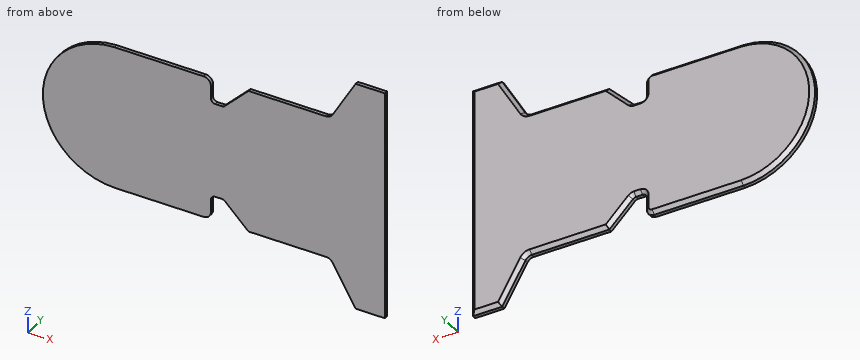
```python
from build123d import *

# Parameters (mm, degrees)
BOSS_EXTRUDE1_DEPTH = 5
CHAMFER1_SIZE       = 2.5


with BuildPart() as part:
    # Sketch1 → Boss-Extrude1 (new body)
    with BuildSketch(Plane(origin=(0, 0, 0), x_dir=(1, 0, 0), z_dir=(0, 1, 0))):
        with BuildLine():
            Line((15.254575611, 35.990242765), (15.254575611, 44.990242765))
            ThreePointArc((15.254575611, 44.990242765), (13.790109517, 48.525776671), (10.254575611, 49.990242765))
            Line((10.254575611, 49.990242765), (-50.745424389, 49.990242765))
            ThreePointArc((-50.745424389, 49.990242765), (-99.757685432, 0), (-50.745424389, -49.990242765))
            Line((-50.745424389, -49.990242765), (10.254575611, -49.990242765))
            ThreePointArc((10.254575611, -49.990242765), (13.790109517, -48.525776671), (15.254575611, -44.990242765))
            Line((15.254575611, -44.990242765), (15.254575611, -35.990242765))
            ThreePointArc((15.254575611, -35.990242765), (16.133255268, -33.868922422), (18.254575611, -32.990242765))
            Line((18.254575611, -32.990242765), (22.711934924, -32.990242765))
            ThreePointArc((22.711934924, -32.990242765), (23.859985221, -33.218604168), (24.833255268, -33.868922422))
            Line((24.833255268, -33.868922422), (40.954575611, -49.990242765))
            Line((40.954575611, -49.990242765), (50.745424389, -49.990242765))
            Line((50.745424389, -49.990242765), (94.067824265, -49.990242765))
            ThreePointArc((94.067824265, -49.990242765), (96.567824265, -50.660115747), (98.397951284, -52.490242765))
            Line((98.397951284, -52.490242765), (114.280717029, -80))
            Line((114.280717029, -80), (134.280717029, -80))
            Line((134.280717029, -80), (134.280717029, 80))
            Line((134.280717029, 80), (114.280717029, 80))
            Line((114.280717029, 80), (98.397951284, 52.490242765))
            ThreePointArc((98.397951284, 52.490242765), (96.567824265, 50.660115747), (94.067824265, 49.990242765))
            Line((94.067824265, 49.990242765), (50.745424389, 49.990242765))
            Line((50.745424389, 49.990242765), (40.954575611, 49.990242765))
            Line((40.954575611, 49.990242765), (24.833255268, 33.868922422))
            ThreePointArc((24.833255268, 33.868922422), (23.859985221, 33.218604168), (22.711934924, 32.990242765))
            Line((22.711934924, 32.990242765), (18.254575611, 32.990242765))
            ThreePointArc((18.254575611, 32.990242765), (16.133255268, 33.868922422), (15.254575611, 35.990242765))
        make_face()
    extrude(amount=BOSS_EXTRUDE1_DEPTH)

    # Chamfer1
    chamfer1_edges = [part.edges().sort_by_distance(p)[0] for p in [
        (96.567824265, 5, 50.660115747),
        (106.339334157, 5, 66.245121383),
        (96.567824265, 5, -50.660115747),
        (124.280717029, 5, 80),
        (134.280717029, 5, 0),
        (124.280717029, 5, -80),
        (67.511199938, 5, -49.990242765),
        (32.893915439, 5, -41.929582594),
        (23.859985221, 5, -33.218604168),
        (20.483255268, 5, -32.990242765),
        (16.133255268, 5, -33.868922422),
        (15.254575611, 5, -40.490242765),
        (13.790109517, 5, -48.525776671),
        (-20.245424389, 5, -49.990242765),
        (-99.757685432, 5, 0),
        (106.339334157, 5, -66.245121383),
        (-20.245424389, 5, 49.990242765),
        (13.790109517, 5, 48.525776671),
        (15.254575611, 5, 40.490242765),
        (16.133255268, 5, 33.868922422),
        (20.483255268, 5, 32.990242765),
        (23.859985221, 5, 33.218604168),
        (32.893915439, 5, 41.929582594),
        (67.511199938, 5, 49.990242765),
    ]]
    chamfer(chamfer1_edges, length=CHAMFER1_SIZE)


solid = part.part
```
Verification items for the finished model (mm, model axes). Coordinates: 2 decimals unless noted, no trailing zeros. Write each loop counter-clockwise with the first axis right and the second up, starting at its lowest first coordinate (ties: lowest second). Pieces come first, ordered by that corner, then holes. Notation, with made-up numbers: M -14,-12.75 L -4,-12.75 A14 cw -4,-0.75 Z; hole C 46.25,89 d11. An arc over 180 degrees is marked long. Answer as a JSON object with one key per item and string values. Group by question number.
(1) Cross-section at C-C, the plane z = 60.5. Record the cut outline in (x, y), and give its area (3 significant figures).
(2) Material ranges on line 1 (Z direction, x = -36, y = 1.35); line 2 (Z direction, x = 18, y = 2.4); line 3 (X direction, y = 1.45, z = -44.5), recorded low to high.
(3) Cross-section at A-A, the plane y = 1.15. Record the cut outline in (x, z), and give its area (3 significant figures).
(4) Cross-section at B-B, the plane x = 1. Record the cut outline in (y, z).
(5) Gauge pin test, flat ends, axial feed: pin 1 (3 mm diameter, centred on x = 19.5, y = 1.5, fed in from -Z); pin 2 (2 mm diameter, centred on x = 20.5, y = 1.5, fed in from +Z); pin 3 (1.2 mm diameter, centred on x = 80.5, y = 0.5, fed in from +Z). Record the tip position at first contact, or that the pin passes through.
Reply:
{
 "1": {"outline": "M 103.02,0 L 134.28,0 L 134.28,2.5 L 131.78,5 L 105.91,5 L 103.02,2.5 Z", "area": "150 mm²"},
 "2": {"line 1": "-49.99 to 49.99", "line 2": "-33 to 33", "line 3": "-72.56 to 15.25, 35.46 to 134.28"},
 "3": {"outline": "M -50.75,-49.99 L 10.25,-49.99 A5 ccw 15.25,-44.99 L 15.25,-35.99 A3 cw 18.25,-32.99 L 22.71,-32.99 A3 cw 24.83,-33.87 L 40.95,-49.99 L 94.07,-49.99 A5 cw 98.4,-52.49 L 114.28,-80 L 134.28,-80 L 134.28,80 L 114.28,80 L 98.4,52.49 A5 cw 94.07,49.99 L 40.95,49.99 L 24.83,33.87 A3 cw 22.71,32.99 L 18.25,32.99 A3 cw 15.25,35.99 L 15.25,44.99 A5 ccw 10.25,49.99 L -50.75,49.99 A50 ccw Z", "area": "23,500 mm²"},
 "4": {"outline": "M 0,-49.99 L 2.5,-49.99 L 5,-47.49 L 5,47.49 L 2.5,49.99 L 0,49.99 Z"},
 "5": {"pin 1": "z = -33", "pin 2": "z = 32.99", "pin 3": "z = 49.99"}
}
